Verification items for the finished model (mm, model axes). A direction names the side the tool comes from. Round coordinates to 2 decimals unless told otherwise and drop trailing zeros. Order: outer loops, then holes, each group sorted by start corner. A loop starts at its lowest first (then second) coordinate and runs counter-clockwise, first axis right, second up.
```python
from build123d import *

# Parameters (mm, degrees)
SKETCH_1_R          = 1.5
SKETCH_1_R_2        = 3
EXTRUDE_1_DEPTH     = 2.5
SKETCH_2_R          = 4.85
EXTRUDE_2_DEPTH     = 4.8
SKETCH_3_R          = 2.925
CUT_EXTRUDE_1_DEPTH = 4.5
SKETCH_4_R          = 1.5
CUT_EXTRUDE_2_DEPTH = 4.5


with BuildPart() as part:
    # 草图1 → 凸台-拉伸1 (new body)
    # profile 1 of 3: a face of its own
    with BuildSketch(Plane.XY):
        with BuildLine():
            Line((-0.710112316, 4.79773285), (-19.7, 3.4))
            ThreePointArc((-19.7, 3.4), (-23.1, 0), (-19.7, -3.4))
            Line((-19.7, -3.4), (-0.710112316, -4.79773285))
            ThreePointArc((-0.710112316, -4.79773285), (-4.85, 0), (-0.710112316, 4.79773285))
        make_face()
        with Locations((-19.7, 0)):
            Circle(SKETCH_1_R, mode=Mode.SUBTRACT)
        with Locations((-15.6, 0)):
            Circle(SKETCH_1_R, mode=Mode.SUBTRACT)
        with Locations((-11.5, 0)):
            Circle(SKETCH_1_R, mode=Mode.SUBTRACT)
    # profile 2 of 3: a face of its own
    with BuildSketch(Plane.XY):
        with BuildLine():
            Line((19.7, 3.4), (0.710112316, 4.79773285))
            ThreePointArc((0.710112316, 4.79773285), (3.671957566, 3.168474023), (4.85, 0))
            ThreePointArc((4.85, 0), (3.671957566, -3.168474023), (0.710112316, -4.79773285))
            Line((0.710112316, -4.79773285), (19.7, -3.4))
            ThreePointArc((19.7, -3.4), (23.1, 0), (19.7, 3.4))
        make_face()
        with Locations((11.5, 0)):
            Circle(SKETCH_1_R, mode=Mode.SUBTRACT)
        with Locations((15.6, 0)):
            Circle(SKETCH_1_R, mode=Mode.SUBTRACT)
        with Locations((19.7, 0)):
            Circle(SKETCH_1_R, mode=Mode.SUBTRACT)
    # profile 3 of 3: a face of its own
    with BuildSketch(Plane.XY):
        with BuildLine():
            Line((0, 4.85), (-0.710112316, 4.79773285))
            ThreePointArc((-0.710112316, 4.79773285), (-4.85, 0), (-0.710112316, -4.79773285))
            Line((-0.710112316, -4.79773285), (0, -4.85))
            Line((0, -4.85), (0.710112316, -4.79773285))
            ThreePointArc((0.710112316, -4.79773285), (3.671957566, -3.168474023), (4.85, 0))
            ThreePointArc((4.85, 0), (3.671957566, 3.168474023), (0.710112316, 4.79773285))
            Line((0.710112316, 4.79773285), (0, 4.85))
        make_face()
        Circle(SKETCH_1_R_2, mode=Mode.SUBTRACT)
    extrude(amount=EXTRUDE_1_DEPTH)

    # 草图2 → 凸台-拉伸2 (add)
    with BuildSketch(Plane.XY.offset(2.5)):
        with Locations(Location((0, 0, 0), (0, 0, 98.419222119))):
            Circle(SKETCH_2_R)
    extrude(amount=EXTRUDE_2_DEPTH)

    # 草图3 → 切除-拉伸1 (cut)
    with BuildSketch(Plane.XY.offset(7.3)):
        Circle(SKETCH_3_R)
    extrude(amount=-CUT_EXTRUDE_1_DEPTH, mode=Mode.SUBTRACT)

    # 草图4 → 切除-拉伸2 (cut)
    with BuildSketch(Plane(origin=(0, 0, 2.5), x_dir=(-1, 0, 0), z_dir=(0, 0, -1))):
        Circle(SKETCH_4_R)
    extrude(amount=-CUT_EXTRUDE_2_DEPTH, mode=Mode.SUBTRACT)


solid = part.part
```
1) Sectioned sample at A-A on x = -11.5. Record the cut outline in (y, z).
2) Sectioned sample at B-B on y = 0. Count the separate pieces of the cut face and the enclosed holes in it, then the cut area to 3 significant figures.
3) Scan lines: probe 1 along Y at (x, z) = (0, 2.7); probe 2 along Y at (x, z) = (0, 5.25) (3 decimals); probe 3 along Z at (x, y) = (-8.5, 2). Record each from-to range of solid material in increasing order.
4) Draft check along Y on faces 4 (the cylindrical face through (-16.8, -0.9, 1.2)), 5 (the cylindrical face through (-0.634, -2.855, 5.082)), 6 (the cylindrical face through (4.838, -0.347, 4.866)), 7 (the flat face through (3.1, 0.4, 7.3)). Enter one of: released by +Y, released by -Y, zero draft, split by the parting line, or undercut.
5) Sectioned sample at C-C on z = 4.5. Record the cut outline in (x, y) (3 decimals), then the cut area to 3 significant figures.
6) Tool access check on faces 1 (the cylindrical face through (-3, 0, 1)), 2 (the flat face through (1.3, -1.3, 2.8)), 3 (the cylindrical face through (-18.27, 0.45, 1.23)). Record the directions out of +Z, -Z, +X, -X, +Y, -Y that give a thin tool (end or side, any length) a straight path to the whole face; none if there is none.
7) Go/stop test with flat-tipped pins: pin 1 Ø1.8 at (x, y) = (11.5, 0) entering from +Z; pin 2 Ø1.8 at (x, y) = (-1, -0.5) entering from -Z; pin 3 Ø4 at (x, y) = (12.5, -1.5) entering from +Z; pin 4 Ø1 at (x, z) = (2, 2) entering from +Y. Record where each tip stops, or that it passes through.
8) Sectioned sample at D-D on x = 15.6. Record the cut outline in (y, z), then the cut area to 3 significant figures.
Returned:
1. outline: (-4, 0) - (-1.5, 0) - (-1.5, 2.5) - (-4, 2.5) - close; (1.5, 0) - (4, 0) - (4, 2.5) - (1.5, 2.5) - close
2. separate pieces: 8
2. enclosed holes: 0
2. area: 74.8 mm2
3. probe 1: y = -4.85 to -1.5, 1.5 to 4.85
3. probe 2: y = -4.85 to -2.925, 2.925 to 4.85
3. probe 3: z = 0 to 2.5
4. face 4: undercut
4. face 5: undercut
4. face 6: split by the parting line
4. face 7: zero draft
5. outline: circle Ø9.7 at (0, 0); hole circle Ø5.85 at (0, 0)
5. area: 47.0 mm2
6. face 1: -Z
6. face 2: +Z
6. face 3: +Z, -Z
7. pin 1: passes through
7. pin 2: stops at z = 2.5
7. pin 3: stops at z = 2.5
7. pin 4: stops at y = 4.74
8. outline: (-3.7, 0) - (-1.5, 0) - (-1.5, 2.5) - (-3.7, 2.5) - close; (1.5, 0) - (3.7, 0) - (3.7, 2.5) - (1.5, 2.5) - close
8. area: 11.0 mm2
